```python
from build123d import *

# Parameters (mm, degrees)
F0_R     = 10
F1_DEPTH = 8


with BuildPart() as f1:
    # F0 (on Top) → F1 (new body)
    with BuildSketch(Plane.XY):
        with BuildLine():
            ThreePointArc((66.8107155763, 68.8983527146), (89.2220086446, 61.1485010982), (103.2801650714, 80.2454771665))
            ThreePointArc((103.2801650714, 80.2454771665), (102.8817929615, 84.2174016446), (101.7025466654, 88.0310957293))
            ThreePointArc((101.7025466654, 88.0310957293), (73.6640874011, 97.7820404055), (66.8107155763, 68.8983527146))
        make_face()
        with Locations((83.2801650714, 80.2454771665)):
            Circle(F0_R, mode=Mode.SUBTRACT)
        with BuildLine():
            ThreePointArc((66.8107155763, 68.8983527146), (73.6640874011, 97.7820404055), (101.7025466654, 88.0310957293))
            Line((101.7025466654, 88.0310957293), (96.8992238213, 99.3967496769))
            ThreePointArc((96.8992238213, 99.3967496769), (71.3236564608, 100.476441104), (59.9351524158, 77.550967172))
            ThreePointArc((59.9351524158, 77.550967172), (63.5204352748, 73.3418677958), (66.8107155763, 68.8983527146))
        make_face()
        with BuildLine():
            ThreePointArc((59.9351524158, 77.550967172), (71.3236564608, 100.476441104), (96.8992238213, 99.3967496769))
            Line((96.8992238213, 99.3967496769), (90.8352022654, 113.7454771665))
            Line((90.8352022654, 113.7454771665), (-90.8352022654, 113.7454771665))
            Line((-90.8352022654, 113.7454771665), (-96.8992238213, 99.3967496769))
            ThreePointArc((-96.8992238213, 99.3967496769), (-72.5051449003, 101.1296563534), (-59.7801650714, 80.2454771665))
            ThreePointArc((-59.7801650714, 80.2454771665), (-59.8189439032, 78.8959953041), (-59.9351524158, 77.550967172))
            ThreePointArc((-59.9351524158, 77.550967172), (0, 104), (59.9351524158, 77.550967172))
        make_face()
        with BuildLine():
            ThreePointArc((-66.8107155763, 68.8983527146), (-63.5204352748, 73.3418677958), (-59.9351524158, 77.550967172))
            ThreePointArc((-59.9351524158, 77.550967172), (-59.8189439032, 78.8959953041), (-59.7801650714, 80.2454771665))
            ThreePointArc((-59.7801650714, 80.2454771665), (-72.5051449003, 101.1296563534), (-96.8992238213, 99.3967496769))
            Line((-96.8992238213, 99.3967496769), (-101.7025466654, 88.0310957293))
            ThreePointArc((-101.7025466654, 88.0310957293), (-79.3082405933, 99.8471050565), (-63.2801650714, 80.2454771665))
            ThreePointArc((-63.2801650714, 80.2454771665), (-64.1831890032, 74.3036335933), (-66.8107155763, 68.8983527146))
        make_face()
        with BuildLine():
            ThreePointArc((-101.7025466654, 88.0310957293), (-92.8962427418, 62.7089139274), (-66.8107155763, 68.8983527146))
            ThreePointArc((-66.8107155763, 68.8983527146), (-64.1831890032, 74.3036335933), (-63.2801650714, 80.2454771665))
            ThreePointArc((-63.2801650714, 80.2454771665), (-79.3082405933, 99.8471050565), (-101.7025466654, 88.0310957293))
        make_face()
        with Locations((-83.2801650714, 80.2454771665)):
            Circle(F0_R, mode=Mode.SUBTRACT)
        Polygon((-90.8352022654, 113.7454771665), (90.8352022654, 113.7454771665), (50, 210.37), (0, 210.37), (-50, 210.37), align=None)
    extrude(amount=F1_DEPTH)


solid = f1.part
```
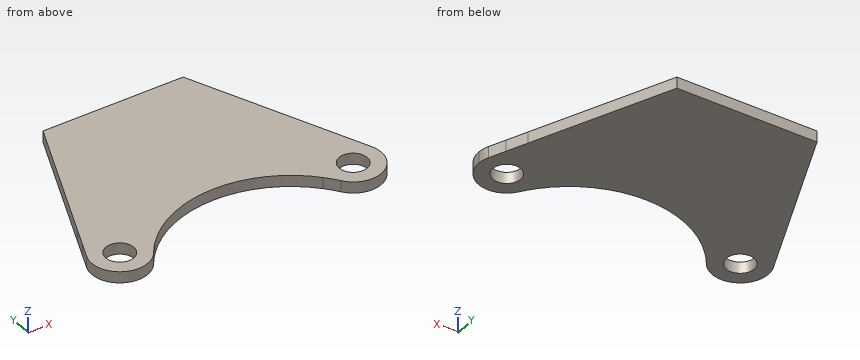
The listing builds one solid part. Answer for the finished solid, in the listing's coordinates (mm). Round coordinates to 2 decimals unless told otherwise and drop trailing zeros. Loops run counter-clockwise (first coordinate to the right, second up) from the corner with the lowest first, then second, coordinate; pieces in that order, holes last. Notation, with made-up numbers: (22, -34) - (57, -34) arc R13 cw to (57, -21) - close; hole circle Ø3 at (39, 72.25). An arc over 180 degrees is marked (long way). Use one line per item in the form item = value. Start each with the question number.
1. The part is cut by section B-B on z = 4.75. Determine the outline of the cut face in (x, y).
2. Consider line 1 (Y direction, x = -80.5, z = 3.25); line 2 (X direction, y = 88, z = 6); line 3 (Y direction, x = 79, z = 5.75). Determine where each line is inside the solid, lowest interval first. Write a range as [from, to].
3. The part is cut by section D-D on y = 142.5. Determine the outline of the cut face in (x, z), then the cut area to 3 significant figures.
4. The part is cut by section C-C on x = 77. Determine the outline of the cut face in (y, z), then the cut area to 3 significant figures.
5. The part is cut by section A-A on y = 75.5. Determine the outline of the cut face in (x, z).
6. Given pin 1 Ø4 at (x, z) = (-64.5, 5) entering from -Y; pin 2 Ø3 at (y, z) = (161.5, 1.5) entering from +X; pin 3 Ø4 at (y, z) = (186, 6) entering from -X; pin 4 Ø23 at (x, y) = (-83.28, 80.25) entering from -Z, each flat-ended and moving along its own axis, determine where each tip first touches the part or whether it passes through.
Geometry check:
q1.outline = (-101.7, 88.03) arc R20 ccw to (-66.81, 68.9) arc R81.13 cw to (66.81, 68.9) arc R20 ccw to (101.7, 88.03) - (50, 210.37) - (-50, 210.37) - close; hole circle Ø20 at (-83.28, 80.25); hole circle Ø20 at (83.28, 80.25)
q2.line_1 = [60.44, 70.64], [89.85, 138.2]
q2.line_2 = [-101.72, -89.59], [-76.97, -48.38], [48.38, 76.97], [89.59, 101.72]
q2.line_3 = [60.71, 71.21], [89.28, 141.75]
q3.outline = (-78.68, 0) - (78.68, 0) - (78.68, 8) - (-78.68, 8) - close
q3.area = 1,260 mm^2
q4.outline = (61.26, 0) - (72.46, 0) - (72.46, 8) - (61.26, 8) - close; (88.03, 0) - (146.48, 0) - (146.48, 8) - (88.03, 8) - close
q4.area = 557 mm^2
q5.outline = (-102.71, 0) - (-92.08, 0) - (-92.08, 8) - (-102.71, 8) - close; (-74.48, 0) - (-61.74, 0) - (-61.74, 8) - (-74.48, 8) - close; (61.74, 0) - (74.48, 0) - (74.48, 8) - (61.74, 8) - close; (92.08, 0) - (102.71, 0) - (102.71, 8) - (92.08, 8) - close
q6.pin_1 = 69.35
q6.pin_2 = 71.29
q6.pin_3 = -61.14
q6.pin_4 = 0
